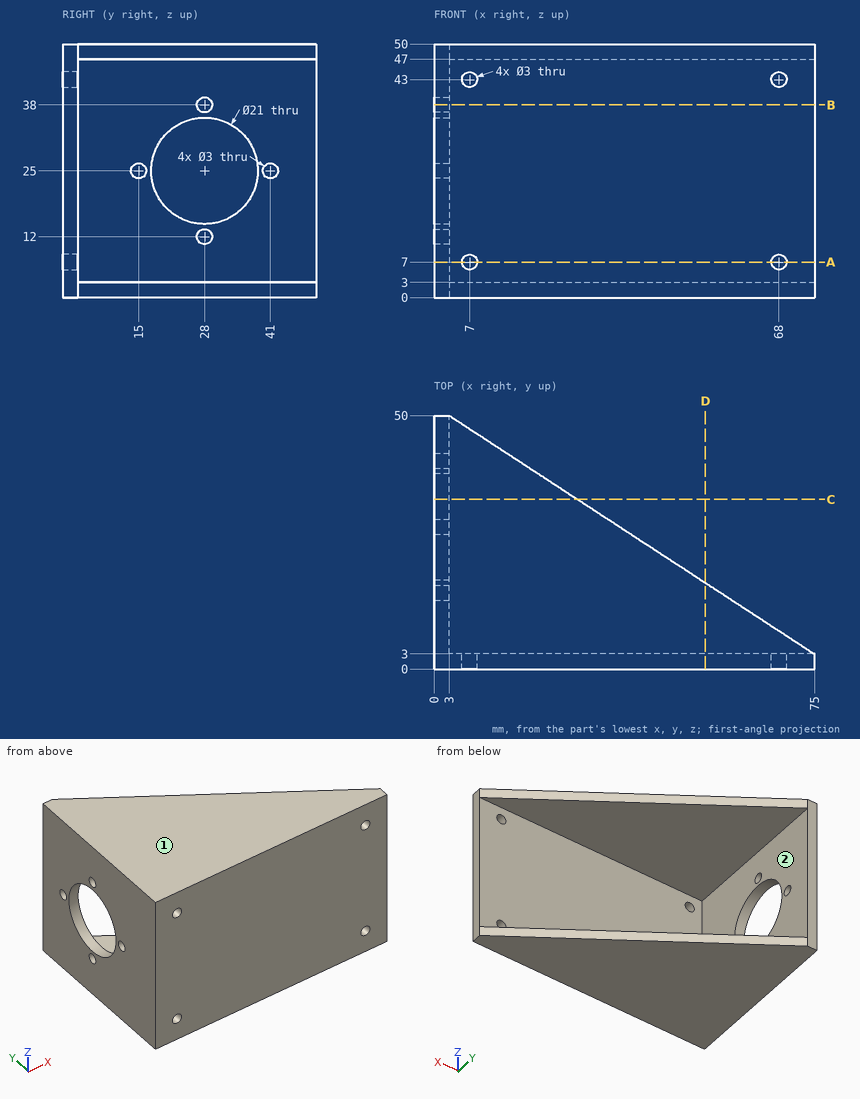
Design review of the part shown in the three views and the two pictorial views. Dimensions are in mm from the part's minimum x, y and z. A direction names the side the tool comes from. Give positions to 0.01 mm unless a question says otherwise; leave off trailing zeros. Write each loop counter-clockwise with the first axis right and the second up, starting at its lowest first coordinate (ties: lowest second). Pieces come first, ordered by that corner, then holes. Notation, with made-up numbers: M 43.5,-27.75 L 77.5,-27.75 A5 ccw 77.5,-18.75 Z; hole C -33,-15.75 d9. An arc over 180 degrees is marked long. One line per question, with ' | ' between items. Start each with the question number.
Item 1: We need section C-C on y = 33.5. Write out the cut boundary in (x, z).
Item 2: For pin 1 (10 mm diameter, centred on x = 66, z = 29, fed in from +Y); pin 2 (5 mm diameter, centred on y = 41, z = 25, fed in from +X), all flat-tipped, find the tip position at first contact; note any pin that passes through.
Item 3: For the marked faces 1 and 2, list the 3-axis set-ups (+Z, -Z, +X, -X, +Y, -Y) from which the entire face can be reached by the end or side of a thin tool; tool diameter is ignored.
Item 4: We need section B-B on z = 38. Write out the cut boundary in (x, y), plus the area to 3 significant figures.
Item 5: We need section D-D on x = 53.5. Write out the cut boundary in (y, z).
Item 6: We need section A-A on z = 7. Write out the cut boundary in (x, y).
Item 7: Wall thickness on line 1 (Z direction, x = 12, y = 29.5); line 2 (Y direction, x = 0.75, z = 38); line 3 (X direction, y = 21, z = 13.5): over which ranges is each line inside the solid? List them lowest first. Write a range as from..to.
Results found:
1) outline: M 0,0 L 28.28,0 L 28.28,3 L 3,3 L 3,16.06 L 0,16.06 Z; M 0,33.94 L 3,33.94 L 3,47 L 28.28,47 L 28.28,50 L 0,50 Z
2) pin 1: stops at y = 3 | pin 2: stops at x = 3
3) face 1: +Z, +X, -X, +Y, -Y | face 2: +X, +Y
4) outline: M 0,0 L 75,0 L 75,3 L 3,3 L 3,26.5 L 0,26.5 Z; M 0,29.5 L 3,29.5 L 3,50 L 0,50 Z | area: 357 mm2
5) outline: M 0,0 L 17.03,0 L 17.03,3 L 3,3 L 3,47 L 17.03,47 L 17.03,50 L 0,50 Z
6) outline: M 0,0 L 5.5,0 L 5.5,3 L 3,3 L 3,50 L 0,50 Z; M 8.5,0 L 66.5,0 L 66.5,3 L 8.5,3 Z; M 69.5,0 L 75,0 L 75,3 L 69.5,3 Z
7) line 1: z = 0..3, 47..50 | line 2: y = 0..26.5, 29.5..50 | line 3: x = 0..3
